Geometry check sheet. Reference: the model listing, model coordinates, mm. A direction names the side the tool comes from. Round coordinates to 2 decimals unless told otherwise and drop trailing zeros. Loops run counter-clockwise (first coordinate to the right, second up) from the corner with the lowest first, then second, coordinate; pieces in that order, holes last. Notation, with made-up numbers: M 29,-0.5 L 66,-0.5 A33 ccw 66,36.5 Z; hole C 69,19 d2. An arc over 180 degrees is marked long. Use one line per item in the form item = value. Start each with the question number.
1. Cross-section at D-D (z = 7). Record the boundary of the cut face in (x, y).
2. Draft check along Y on faces 1 (the flat face through (-7, 15, 44)), 2 (the flat face through (-22, 0, 31)), 3 (the cylindrical face through (197.15, 246.05, 31.31)). Enter one of: pulls with the +Y half, pulls with the -Y half, needs draft (parallel to the pull), parting line crosses it, or undercut.
3. Go/stop test with flat-tipped pins: pin 1 (1 mm diameter, centred on y = 113.5, z = 12, fed in from +X); pin 2 (1 mm diameter, centred on y = 48.5, z = 55.5, fed in from -X); pin 3 (11.5 mm diameter, centred on y = 137.5, z = 50, fed in from +X). Record where each tip stops, or that it passes through.
4. Cross-section at C-C (y = 125). Record the boundary of the cut face in (x, z), then the cut area to 3 significant figures.
5. Material ranges on line 1 (Y direction, x = 165.5, z = 38); line 2 (X direction, y = 124, z = 40.5); line 3 (X direction, y = 94, z = 37), recorded low to high.
6. Cross-section at B-B (x = -50.5). Record the boundary of the cut face in (y, z), then the cut area to 3 significant figures.
7. Set-up check for faces 4 (the flat face through (-17, 250, 31)), 5 (the flat face through (-7, 127, 25.4)): record each of +Z, -Z, +X, -X, +Y, -Y from which the full face is reachable in a straight line by a thin tool's end or side.
8. Cross-section at A-A (z = 34). Record the boundary of the cut face in (x, y), then the cut area to 3 significant figures.
```python
from build123d import *

# Parameters (mm, degrees)
F1_DEPTH = 25.4
F2_W     = 396.535074
F2_H     = 220
F3_DEPTH = 38.1
F4_R     = 177.372541
F5_R     = 149.724354
F6_R     = 177.3682
F7_R     = 149.733


with BuildPart() as f1:
    # F0 (on Top) → F1 (new body)
    with BuildSketch(Plane.XY):
        with BuildLine():
            ThreePointArc((-202.424236, 250), (-327.424236, 125), (-202.424236, 0))
            Line((-202.424236, 0), (197.575764, 0))
            Line((197.575764, 0), (296.114177, 48.089784))
            ThreePointArc((296.114177, 48.089784), (376.654646, 125), (296.114177, 201.910216))
            Line((296.114177, 201.910216), (197.575764, 250))
            Line((197.575764, 250), (-202.424236, 250))
        make_face()
    extrude(amount=F1_DEPTH)

    # F2 (on face) → F3 (join)
    with BuildSketch(Plane.XY.offset(25.4)):
        with BuildLine():
            Line((197.575764, 250), (-202.424236, 250))
            ThreePointArc((-202.424236, 250), (-327.424236, 125), (-202.424236, 0))
            Line((-202.424236, 0), (197.575764, 0))
            Line((197.575764, 0), (296.114177, 48.089784))
            ThreePointArc((296.114177, 48.089784), (376.654646, 125), (296.114177, 201.910216))
            Line((296.114177, 201.910216), (197.575764, 250))
        make_face()
        with Locations((-4.156699, 125)):
            Rectangle(F2_W, F2_H, mode=Mode.SUBTRACT)
    extrude(amount=F3_DEPTH)

    # F4
    f4_edges = [f1.edges().sort_by_distance(p)[0] for p in [
        (296.114177, 201.910216, 31.75),
    ]]
    fillet(f4_edges, radius=F4_R)

    # F5
    f5_edges = [f1.edges().sort_by_distance(p)[0] for p in [
        (197.575764, 250, 31.75),
    ]]
    fillet(f5_edges, radius=F5_R)

    # F6
    f6_edges = [f1.edges().sort_by_distance(p)[0] for p in [
        (296.114177, 48.089784, 31.75),
    ]]
    fillet(f6_edges, radius=F6_R)

    # F7
    f7_edges = [f1.edges().sort_by_distance(p)[0] for p in [
        (197.575764, 0, 31.75),
    ]]
    fillet(f7_edges, radius=F7_R)


solid = f1.part
```
Reported:
q1.outline = M -202.42,0 L 162.99,0 A149.73 ccw 228.66,15.17 L 267.63,34.19 A177.37 cw 313.51,49.26 A76.99 ccw 313.51,200.74 A177.37 cw 267.63,215.81 L 228.66,234.83 A149.72 ccw 162.99,250 L -202.42,250 A125 ccw Z
q2.face_1 = undercut
q2.face_2 = pulls with the -Y half
q2.face_3 = pulls with the +Y half
q3.pin_1 = 375.86
q3.pin_2 = -301.67
q3.pin_3 = 376.36
q4.outline = M -327.42,0 L 376.65,0 L 376.65,63.5 L 194.11,63.5 L 194.11,25.4 L -202.42,25.4 L -202.42,63.5 L -327.42,63.5 Z
q4.area = 29,600 mm²
q5.line_1 = 0.02 to 15, 235 to 249.98
q5.line_2 = -327.42 to -202.42, 194.11 to 376.65
q5.line_3 = -323.52 to -202.42, 194.11 to 370.14
q6.outline = M 0,0 L 250,0 L 250,63.5 L 235,63.5 L 235,25.4 L 15,25.4 L 15,63.5 L 0,63.5 Z
q6.area = 7,490 mm²
q7.face_4 = +Z, -Z, +X, -X, +Y
q7.face_5 = +Z
q8.outline = M -202.42,0 L 162.99,0 A149.73 ccw 228.66,15.17 L 267.63,34.19 A177.37 cw 313.51,49.26 A76.99 ccw 313.51,200.74 A177.37 cw 267.63,215.81 L 228.66,234.83 A149.72 ccw 162.99,250 L -202.42,250 A125 ccw Z; hole M -202.42,15 L 194.11,15 L 194.11,235 L -202.42,235 Z
q8.area = 67,000 mm²
